```python
from build123d import *

# Parameters (mm, degrees)
SKETCH_3_W             = 0.1
SKETCH_3_H             = 7.8
SKETCH_3_W_2           = 8
EXTRUDE_1_DEPTH        = 7.4
CUT_EXTRUDE_1_REACH    = 22.97
SKETCH_4_R             = 2.5
SKETCH_4_3_R           = 3.15
SKETCH_4_3_R_2         = 2.5
CUT_EXTRUDE_2_DEPTH    = 1
CUT_EXTRUDE_START      = -6.8
SKETCH_4_4_R           = 3.15
SKETCH_4_4_R_2         = 2.5
CUT_EXTRUDE_3_DEPTH    = 1
SKETCH_5_R             = 2.5
CUT_EXTRUDE_4_DEPTH    = 26.844341741
SKETCH_5_3_R           = 3.15
SKETCH_5_3_R_2         = 2.5
CUT_EXTRUDE_5_DEPTH    = 1
SKETCH_5_4_R           = 3.15
SKETCH_5_4_R_2         = 2.5
CUT_EXTRUDE_6_DEPTH    = 1
CUT_EXTRUDE_9_DEPTH    = 2
CUT_EXTRUDE_START_2    = -5.8
CUT_EXTRUDE_10_DEPTH   = 2
PATTERN_LINEAR_1_COUNT = 2
PATTERN_LINEAR_1_PITCH = 8
SKETCH_7_W             = 7.95
SKETCH_7_H             = 7.8
EXTRUDE_2_DEPTH        = 7.8
PATTERN_LINEAR_2_COUNT = 2
PATTERN_LINEAR_2_PITCH = 8
CUT_EXTRUDE_11_DEPTH   = 2
CUT_EXTRUDE_12_DEPTH   = 2
FILLET_1_R             = 3.5


with BuildPart() as part:
    # 草图3 → 凸台-拉伸1 (new body)
    with BuildSketch(Plane(origin=(0, 0, 0), x_dir=(0, 0, -1), z_dir=(1, 0, 0))):
        with Locations((-4.05, 3.9)):
            Rectangle(SKETCH_3_W, SKETCH_3_H)
        Polygon((-11.9, 0), (-4.1, 0), (-4.1, 7.8), (-4.1, 23.4), (-11.9, 23.4), align=None)
        with Locations((0, 3.9)):
            Rectangle(SKETCH_3_W_2, SKETCH_3_H)
    extrude(amount=EXTRUDE_1_DEPTH)

    # 草图4 → 切除-拉伸1 (cut, up to next)
    with BuildSketch(Plane(origin=(0, 7.8, 0), x_dir=(1, 0, 0), z_dir=(0, 1, 0)), mode=Mode.PRIVATE) as cut_extrude_1_sk1:
        with Locations(Location((3.7, -0.05, 0), (0, 0, 270))):
            Circle(SKETCH_4_R)
    cut_extrude_1_tool1 = extrude(cut_extrude_1_sk1.sketch, amount=-CUT_EXTRUDE_1_REACH, mode=Mode.PRIVATE) & part.part
    cut_extrude_1 = cut_extrude_1_tool1.solids().sort_by_distance((3.7, 7.8, 0.05))[0]
    add(cut_extrude_1, mode=Mode.SUBTRACT)

    # 草图4<3> → 切除-拉伸2 (cut)
    with BuildSketch(Plane(origin=(0, 7.8, 0), x_dir=(1, 0, 0), z_dir=(0, 1, 0))):
        with Locations(Location((3.7, -0.05, 0), (0, 0, 270))):
            Circle(SKETCH_4_3_R)
        with Locations(Location((3.7, -0.05, 0), (0, 0, 270))):
            Circle(SKETCH_4_3_R_2, mode=Mode.SUBTRACT)
    cut_extrude_2 = extrude(amount=-CUT_EXTRUDE_2_DEPTH, mode=Mode.SUBTRACT)

    # 草图4<4> → 切除-拉伸3 (cut)
    with BuildSketch(Plane(origin=(0, 7.8, 0), x_dir=(1, 0, 0), z_dir=(0, 1, 0)).offset(CUT_EXTRUDE_START)):
        with Locations(Location((3.7, -0.05, 0), (0, 0, 270))):
            Circle(SKETCH_4_4_R)
        with Locations(Location((3.7, -0.05, 0), (0, 0, 270))):
            Circle(SKETCH_4_4_R_2, mode=Mode.SUBTRACT)
    cut_extrude_3 = extrude(amount=-CUT_EXTRUDE_3_DEPTH, mode=Mode.SUBTRACT)

    # 草图5 → 切除-拉伸4 (cut, through all)
    with BuildSketch(Plane(origin=(0, 0, 4.1), x_dir=(-1, 0, 0), z_dir=(0, 0, -1))):
        with Locations(Location((-3.7, 11.7, 0), (0, 0, 90))):
            Circle(SKETCH_5_R)
    cut_extrude_4 = extrude(amount=-CUT_EXTRUDE_4_DEPTH, mode=Mode.SUBTRACT)

    # 草图5<3> → 切除-拉伸5 (cut)
    with BuildSketch(Plane(origin=(0, 0, 4.1), x_dir=(-1, 0, 0), z_dir=(0, 0, -1))):
        with Locations(Location((-3.7, 11.7, 0), (0, 0, 90))):
            Circle(SKETCH_5_3_R)
        with Locations(Location((-3.7, 11.7, 0), (0, 0, 90))):
            Circle(SKETCH_5_3_R_2, mode=Mode.SUBTRACT)
    cut_extrude_5 = extrude(amount=-CUT_EXTRUDE_5_DEPTH, mode=Mode.SUBTRACT)

    # 草图5<4> → 切除-拉伸6 (cut)
    with BuildSketch(Plane(origin=(0, 0, 4.1), x_dir=(-1, 0, 0), z_dir=(0, 0, -1)).offset(CUT_EXTRUDE_START)):
        with Locations(Location((-3.7, 11.7, 0), (0, 0, 90))):
            Circle(SKETCH_5_4_R)
        with Locations(Location((-3.7, 11.7, 0), (0, 0, 90))):
            Circle(SKETCH_5_4_R_2, mode=Mode.SUBTRACT)
    cut_extrude_6 = extrude(amount=-CUT_EXTRUDE_6_DEPTH, mode=Mode.SUBTRACT)

    # 草图6 → 切除-拉伸9 (cut)
    with BuildSketch(Plane(origin=(0, 0, 4.1), x_dir=(-1, 0, 0), z_dir=(0, 0, -1))):
        with BuildLine():
            ThreePointArc((-6.525, 14.089429848), (-3.7, 15.4), (-0.875, 14.089429848))
            Line((-0.875, 14.089429848), (-0.875, 17.310570152))
            ThreePointArc((-0.875, 17.310570152), (-3.7, 16), (-6.525, 17.310570152))
            Line((-6.525, 17.310570152), (-6.525, 14.089429848))
        make_face()
    extrude(amount=-CUT_EXTRUDE_9_DEPTH, mode=Mode.SUBTRACT)

    # 草图6<3> → 切除-拉伸10 (cut)
    with BuildSketch(Plane(origin=(0, 0, 4.1), x_dir=(-1, 0, 0), z_dir=(0, 0, -1)).offset(CUT_EXTRUDE_START_2)):
        with BuildLine():
            ThreePointArc((-6.525, 14.089429848), (-3.7, 15.4), (-0.875, 14.089429848))
            Line((-0.875, 14.089429848), (-0.875, 17.310570152))
            ThreePointArc((-0.875, 17.310570152), (-3.7, 16), (-6.525, 17.310570152))
            Line((-6.525, 17.310570152), (-6.525, 14.089429848))
        make_face()
    extrude(amount=-CUT_EXTRUDE_10_DEPTH, mode=Mode.SUBTRACT)

    # 阵列(线性)1: 切除-拉伸4, 切除-拉伸5, 切除-拉伸6 ×2
    with Locations(*[(0, i * PATTERN_LINEAR_1_PITCH, 0) for i in range(1, PATTERN_LINEAR_1_COUNT)]):
        add(cut_extrude_4, mode=Mode.SUBTRACT)
        add(cut_extrude_5, mode=Mode.SUBTRACT)
        add(cut_extrude_6, mode=Mode.SUBTRACT)

    # 草图7 → 凸台-拉伸2 (add)
    with BuildSketch(Plane(origin=(0, 0, 0), x_dir=(0, 0, -1), z_dir=(1, 0, 0))):
        with Locations((0.025, 3.9)):
            Rectangle(SKETCH_7_W, SKETCH_7_H)
    extrude(amount=-EXTRUDE_2_DEPTH)

    # 阵列(线性)2: 切除-拉伸1, 切除-拉伸2, 切除-拉伸3 ×2
    with Locations(*[(-i * PATTERN_LINEAR_2_PITCH, 0, 0) for i in range(1, PATTERN_LINEAR_2_COUNT)]):
        add(cut_extrude_1, mode=Mode.SUBTRACT)
        add(cut_extrude_2, mode=Mode.SUBTRACT)
        add(cut_extrude_3, mode=Mode.SUBTRACT)

    # 草图9 → 切除-拉伸11 (cut)
    with BuildSketch(Plane.XZ):
        with BuildLine():
            ThreePointArc((0, 0.05), (0.343596386, 1.607098192), (1.310570152, 2.875))
            Line((1.310570152, 2.875), (-1.910570152, 2.875))
            ThreePointArc((-1.910570152, 2.875), (-0.943596386, 1.607098192), (-0.6, 0.05))
            Line((-0.6, 0.05), (0, 0.05))
        make_face()
        with BuildLine():
            Line((-1.910570152, -2.775), (1.310570152, -2.775))
            ThreePointArc((1.310570152, -2.775), (0.343596386, -1.507098192), (0, 0.05))
            Line((0, 0.05), (-0.6, 0.05))
            ThreePointArc((-0.6, 0.05), (-0.943596386, -1.507098192), (-1.910570152, -2.775))
        make_face()
    extrude(amount=-CUT_EXTRUDE_11_DEPTH, mode=Mode.SUBTRACT)

    # 草图9<3> → 切除-拉伸12 (cut)
    with BuildSketch(Plane.XZ.offset(CUT_EXTRUDE_START_2)):
        with BuildLine():
            ThreePointArc((0, 0.05), (0.343596386, 1.607098192), (1.310570152, 2.875))
            Line((1.310570152, 2.875), (-1.910570152, 2.875))
            ThreePointArc((-1.910570152, 2.875), (-0.943596386, 1.607098192), (-0.6, 0.05))
            Line((-0.6, 0.05), (0, 0.05))
        make_face()
        with BuildLine():
            Line((-1.910570152, -2.775), (1.310570152, -2.775))
            ThreePointArc((1.310570152, -2.775), (0.343596386, -1.507098192), (0, 0.05))
            Line((0, 0.05), (-0.6, 0.05))
            ThreePointArc((-0.6, 0.05), (-0.943596386, -1.507098192), (-1.910570152, -2.775))
        make_face()
    extrude(amount=-CUT_EXTRUDE_12_DEPTH, mode=Mode.SUBTRACT)

    # 圆角1
    fillet_1_edges = [part.edges().sort_by_distance(p)[0] for p in [
        (7.4, 23.4, 8),
        (0, 23.4, 8),
        (-7.8, 3.9, -4),
        (-7.8, 3.9, 3.95),
        (3.7, 0, 11.9),
        (7.4, 3.9, -4),
    ]]
    fillet(fillet_1_edges, radius=FILLET_1_R)


solid = part.part
```
Geometry check sheet. Reference: the model listing, model coordinates, mm. A direction names the side the tool comes from. Round coordinates to 2 decimals unless told otherwise and drop trailing zeros. Loops run counter-clockwise (first coordinate to the right, second up) from the corner with the lowest first, then second, coordinate; pieces in that order, holes last. Notation, with made-up numbers: M 69,83 L 82,83 A24 cw 82,100 Z; hole C 43,-25.5 d9. An arc over 180 degrees is marked long. Return JSON: item names as keys, results as strings. Group by question number.
(1) Scan lines: line 1 along X through (y, z) = (11.7, 8.9); line 2 along Y through (x, z) = (-3.25, -2.25); line 3 along X through (y, z) = (11.7, 11.2). Record each from-to range of solid material in increasing order. Write a range as [from, to].
(2) Section check C-C, the plane z = 7. Enter the section's corners in (x, y).
(3) Go/stop test with flat-tipped pins: pin 1 (1.9 mm diameter, centred on x = -5, z = -1.5, fed in from +Y); pin 2 (2.5 mm diameter, centred on x = 0.5, z = -1.5, fed in from +Y); pin 3 (5.5 mm diameter, centred on x = 3.7, z = 0.05, fed in from -Y). Record where each tip stops, or that it passes through.
(4) Section check A-A, the plane z = 10.5. Enter the section's corners in (x, y) (3 decimals), and give its area (3 significant figures).
(5) Mould release check, pull along Z, two halves, no side actions. Record for faces 1 (the face through (-0.3, 5.8, 0.1)), 2 (the face through (3.7, 15.7, 9.9)), 3 (the face through (0, 1, 2.875)), 4 (the face through (1, 14, 4.1)): pulls with the +Z half, pulls with the -Z half, needs draft (parallel to the pull), parting line crosses it, or undercut.
(6) Section check B-B, the plane y = 11.7. Enter the section's corners in (x, z).
(7) Section check D-D, the plane x = -6.5. Enter the section's corners in (y, z).
(8) Set-up check for faces 5 (the face through (0.625, 0.507, -0.633)), 6 (the face through (2.49, 14.61, 4.59)), 7 (the face through (6, 10, 10.9)): record each of +Z, -Z, +X, -X, +Y, -Y from which the full face is reachable in a straight line by a thin tool's end or side.
Data:
{
 "1": {"line 1": "[0, 1.2], [6.2, 7.4]", "line 2": "[1, 6.8]", "line 3": "[0, 0.55], [6.85, 7.4]"},
 "2": {"outline": "M 0,0 L 7.4,0 L 7.4,19.9 A3.5 ccw 3.9,23.4 L 3.5,23.4 A3.5 ccw 0,19.9 Z; hole C 3.7,11.7 d5; hole C 3.7,19.7 d5"},
 "3": {"pin 1": "y = 6.8", "pin 2": "y = 7.8", "pin 3": "y = 1"},
 "4": {"outline": "M 0,0.7 L 7.4,0.7 L 7.4,19.9 A3.5 ccw 3.9,23.4 L 3.5,23.4 A3.5 ccw 0,19.9 Z; hole M 0.875,14.089 A3.7 cw 6.525,14.089 L 6.525,17.311 A3.7 cw 0.875,17.311 Z; hole C 3.7,11.7 d5; hole C 3.7,19.7 d5", "area": "116 mm²"},
 "5": {"face 1": "undercut", "face 2": "pulls with the +Z half", "face 3": "undercut", "face 4": "pulls with the -Z half"},
 "6": {"outline": "M 0,4.1 L 0.55,4.1 L 0.55,5.1 L 1.2,5.1 L 1.2,10.9 L 0.55,10.9 L 0.55,11.9 L 0,11.9 Z; M 6.2,5.1 L 6.85,5.1 L 6.85,4.1 L 7.4,4.1 L 7.4,11.9 L 6.85,11.9 L 6.85,10.9 L 6.2,10.9 Z"},
 "7": {"outline": "M 0,-3.22 L 7.8,-3.22 L 7.8,-2.2 L 6.8,-2.2 L 6.8,-1.14 L 1,-1.14 L 1,-2.2 L 0,-2.2 Z; M 0,2.3 L 1,2.3 L 1,1.24 L 6.8,1.24 L 6.8,2.3 L 7.8,2.3 L 7.8,3.17 L 0,3.17 Z"},
 "8": {"face 5": "-Y", "face 6": "-Z", "face 7": "+Z"}
}
